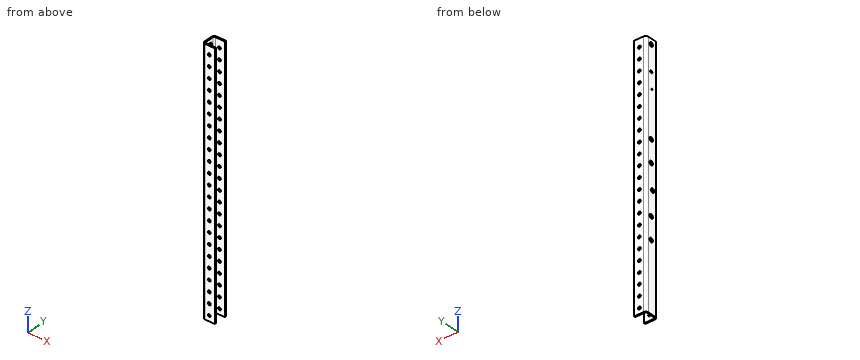
Autodesk Inventor part; units mm, degrees
ref_plane "YZ Plane" through (0, 0, 0) normal (1, 0, 0) x (0, 1, 0)
ref_plane "XZ Plane" through (0, 0, 0) normal (0, 1, 0) x (-1, 0, 0)
ref_plane "XY Plane" through (0, 0, 0) normal (0, 0, 1) x (1, 0, 0)
sketch "Sketch1" plane through (0, 0, 0) normal (0, 0, 1) x (1, 0, 0)
  line L0 (5.9771, 0) -> (28.2021, 0)
  line L1 (28.2021, 0) -> (28.2021, 3.175)
  line L2 (28.2021, 3.175) -> (5.9771, 3.175)
  line L3 (2.8021, 6.35) -> (2.8021, 25.4)
  line L4 (5.9771, 28.575) -> (28.2021, 28.575)
  line L5 (28.2021, 28.575) -> (28.2021, 31.75)
  line L6 (28.2021, 31.75) -> (5.9771, 31.75)
  line L7 (-0.3729, 25.4) -> (-0.3729, 6.35)
  arc A0 (5.9771, 28.575) -> (2.8021, 25.4) centre (5.9771, 25.4) ccw
  arc A1 (2.8021, 6.35) -> (5.9771, 3.175) centre (5.9771, 6.35) ccw
  arc A2 (5.9771, 31.75) -> (-0.3729, 25.4) centre (5.9771, 25.4) ccw
  arc A3 (-0.3729, 6.35) -> (5.9771, 0) centre (5.9771, 6.35) ccw
  point P0 (0, 0)
  point P1 (-0.3729, 0)
  point P2 (2.8021, 3.175)
  point P3 (2.8021, 28.575)
  dimension "d0" = 28.575
  dimension "d1" = 3.175
  dimension "d2" = 25.4
  dimension "d3" = 25.4
  dimension "d4" = 3.175
  dimension "d5" = 3.175
  dimension "d6" = 6.35
extrude "Extrusion1" add sketch "Sketch1" against normal blind 889
sketch "Sketch2" plane through (-0.3729, 6.35, 0) normal (-1, 0, 0) x (0, 0, 1)
  line L0 (0, 19.05) -> (-889, 19.05)
  line L1 (-228.6, 0) -> (-228.6, 7.9375)
  arc A0 (-228.6, 11.1125) -> (-228.6, 7.9375) centre (-228.6, 9.525) ccw
  line L2 (-228.6, 11.1125) -> (-228.6, 19.05)
  line L3 (-228.6, 19.05) -> (-889, 19.05)
  line L4 (-889, 0) -> (-889, 19.05)
  line L5 (-889, 0) -> (-228.6, 0)
  circle A1 centre (-552.45, 11.43) radius 4.826
  circle A2 centre (-501.65, 11.43) radius 4.826
  circle A3 centre (-387.35, 11.43) radius 4.826
  circle A4 centre (-336.55, 11.43) radius 4.826
  circle A5 centre (-444.5, 7.62) radius 4.826
  circle A6 centre (-730.25, 11.43) radius 4.826
  circle A7 centre (-781.05, 11.43) radius 4.826
  line L6 (0, 25.4) -> (-889, 25.4) construction
  circle A8 centre (-133.35, 11.43) radius 4.826
  circle A9 centre (-82.55, 11.43) radius 4.826
  point P0 (0, -6.35)
  point P1 (-254, 0.852)
  dimension "d10" = 7.62
  dimension "d11" = 3.81
  dimension "d14" = 254
hole "Hole1" at (-0.3729, 17.78, -781.05) at (-0.3729, 17.78, -730.25) at (-0.3729, 17.78, -552.45) at (-0.3729, 17.78, -501.65) at (-0.3729, 13.97, -444.5) at (-0.3729, 17.78, -387.35) at (-0.3729, 17.78, -336.55) at (-0.3729, 17.78, -133.35) at (-0.3729, 17.78, -82.55) direction (1, 0, 0) diameter 9.652 end through all
hole "Hole2" at (-0.3729, 15.875, -228.6) direction (1, 0, 0) diameter 3.175 end through all
sketch "Sketch3" plane through (5.9771, 31.75, 0) normal (0, 1, 0) x (1, 0, 0)
  line L0 (22.225, 889) -> (0, 889)
  line L1 (22.225, 0) -> (22.225, 889)
  point P0 (-5.9771, 0)
  point P1 (9.525, 876.3)
  dimension "d34" = 12.7
  dimension "d35" = 12.7
hole "Hole3" at (15.5021, 31.75, -876.3) direction (0, -1, 0) diameter 6.5278 end through all
pattern_linear "Rectangular Pattern1" count 35 spacing 25.4 along (0, 0, 1) of "Hole3"
sketch "Sketch4" plane through (0, 0, 0) normal (0, 0, 1) x (1, 0, 0)
  line L0 (28.2021, 0) -> (5.9771, 0)
  line L1 (28.2021, 3.175) -> (28.2021, 0)
  line L2 (5.9771, 3.175) -> (28.2021, 3.175)
  arc A0 (2.8021, 6.35) -> (5.9771, 3.175) centre (5.9771, 6.35) ccw
  line L3 (2.8021, 25.4) -> (2.8021, 6.35)
  arc A1 (5.9771, 28.575) -> (2.8021, 25.4) centre (5.9771, 25.4) ccw
  line L4 (28.2021, 28.575) -> (5.9771, 28.575)
  line L5 (28.2021, 31.75) -> (28.2021, 28.575)
  line L6 (5.9771, 31.75) -> (28.2021, 31.75)
  arc A2 (5.9771, 31.75) -> (-0.3729, 25.4) centre (5.9771, 25.4) ccw
  line L7 (-0.3729, 6.35) -> (-0.3729, 25.4)
  arc A3 (-0.3729, 6.35) -> (5.9771, 0) centre (5.9771, 6.35) ccw
  point P0 (0, 0)
extrude "Extrusion2" cut sketch "Sketch4" against normal blind 120.65
sketch "Sketch5" plane through (0, 0, -889) normal (0, 0, -1) x (-1, 0, 0)
  line L0 (-28.2021, 0) -> (-28.2021, 3.175)
  line L1 (-5.9771, 0) -> (-28.2021, 0)
  arc A0 (-5.9771, 0) -> (0.3729, 6.35) centre (-5.9771, 6.35) ccw
  line L2 (0.3729, 25.4) -> (0.3729, 6.35)
  arc A1 (0.3729, 25.4) -> (-5.9771, 31.75) centre (-5.9771, 25.4) ccw
  line L3 (-28.2021, 31.75) -> (-5.9771, 31.75)
  line L4 (-28.2021, 28.575) -> (-28.2021, 31.75)
  line L5 (-5.9771, 28.575) -> (-28.2021, 28.575)
  arc A2 (-2.8021, 25.4) -> (-5.9771, 28.575) centre (-5.9771, 25.4) ccw
  line L6 (-2.8021, 6.35) -> (-2.8021, 25.4)
  arc A3 (-5.9771, 3.175) -> (-2.8021, 6.35) centre (-5.9771, 6.35) ccw
  line L7 (-28.2021, 3.175) -> (-5.9771, 3.175)
  point P0 (0, 0)
extrude "Extrusion3" cut sketch "Sketch5" against normal blind 177.8
sketch "Sketch6" plane through (2.8021, 6.35, -120.65) normal (1, 0, 0) x (0, 0, -1)
  circle A0 centre (41.91, 11.43) radius 34.925 construction
  circle A1 centre (21.2554, -9.2246) radius 3.175 construction
  circle A2 centre (12.7, 11.43) radius 3.175 construction
  circle A3 centre (21.2554, 32.0846) radius 3.175 construction
  circle A4 centre (41.91, 40.64) radius 3.175 construction
  circle A5 centre (62.5646, 32.0846) radius 3.175 construction
  circle A6 centre (71.12, 11.43) radius 3.175
  circle A7 centre (62.5646, -9.2246) radius 3.175 construction
  circle A8 centre (41.91, -17.78) radius 3.175 construction
  circle A9 centre (41.91, 11.43) radius 22.86 construction
  point P0 (-120.65, -6.35)
extrude "Extrusion4" cut sketch "Sketch6" against normal through all
properties part number "Center of Mass Shifter Arm - Chassis_Channel_AndyMark"
CAD build for the part. Positions are in the model's coordinates, mm. Coordinates: 2 decimals unless noted, no trailing zeros. Order: outer loops, then holes, each group sorted by start corner. A loop starts at its lowest first (then second) coordinate and runs counter-clockwise, first axis right, second up. Notation, with made-up numbers: (51, 23) -> (77, 23) arc R10 ccw to (77, 35) -> close; hole circle Ø10 at (63, 47.5). An arc over 180 degrees is marked (long way). Answer in a Markdown table with one row per item.
1) Flat gauge pins, fed straight in: P1, Ø3, axis at y = 10.5, z = -349.5, coming from the +X side; P2, Ø6, axis at x = 15.5, z = -571.5, coming from the +Y side. Where does each tip first touch, or does it go through?
Check values:
| item | result |
|---|---|
| P1 | x = 2.8 |
| P2 | through |
2) Drill centre lines: line 1 (Y direction, x = 21.25, z = -502.5) (3 decimals); line 2 (X direction, y = 23, z = -147); line 3 (Y direction, x = 2.75, z = -548). Where is each one in solid material? Low to high.
Check values:
| item | result |
|---|---|
| line 1 | 0 to 3.175, 28.575 to 31.75 |
| line 2 | -0.37 to 2.8 |
| line 3 | 0.88 to 15.91, 19.65 to 30.87 |
3) Band-saw the part on A-A (z = -201.5). List the corners of the cut face in (x, y) (3 decimals), and give its area (3 significant figures).
Check values:
| item | result |
|---|---|
| outline | (-0.373, 6.35) arc R6.35 ccw to (5.977, 0) -> (28.202, 0) -> (28.202, 3.175) -> (5.977, 3.175) arc R3.175 cw to (2.802, 6.35) -> (2.802, 25.4) arc R3.175 cw to (5.977, 28.575) -> (28.202, 28.575) -> (28.202, 31.75) -> (5.977, 31.75) arc R6.35 ccw to (-0.373, 25.4) -> close |
| area | 249 mm2 |
